Could you check a few things on this model? Use its own coordinates, in mm. A direction names the side the tool comes from. Give positions to 0.01 mm unless a question says otherwise; leave off trailing zeros. Write each loop counter-clockwise with the first axis right and the second up, starting at its lowest first coordinate (ties: lowest second). Pieces come first, ordered by that corner, then holes. Notation, with made-up numbers: (4, 37.25) -> (28, 37.25) arc R23 ccw to (28, 67.25) -> close; hole circle Ø7 at (23.25, 13.25). An arc over 180 degrees is marked (long way). Write item = value, one per line. Start each with the question number.
```python
from build123d import *

# Parameters (mm, degrees)
SKETCH1_W                                           = 97
SKETCH1_H                                           = 32.5
BOSS_EXTRUDE1_DEPTH                                 = 6
SKETCH5_R                                           = 20
BOSS_EXTRUDE5_DEPTH                                 = 20
CBORE_FOR_M5_HEX_SOCKET_HEAD_CAP_SCREW1_D           = 5.5
CBORE_FOR_M5_HEX_SOCKET_HEAD_CAP_SCREW1_CBORE_D     = 10
CBORE_FOR_M5_HEX_SOCKET_HEAD_CAP_SCREW1_CBORE_DEPTH = 5.9
SKETCH16_R                                          = 2.5
BOSS_EXTRUDE6_DEPTH                                 = 5
BOSS_EXTRUDE7_START                                 = -27.5
SKETCH16_2_R                                        = 2.5
BOSS_EXTRUDE7_DEPTH                                 = 5
SKETCH17_R                                          = 5
CUT_EXTRUDE3_DEPTH                                  = 3
SKETCH18_R                                          = 5
SKETCH18_R_2                                        = 2.75
BOSS_EXTRUDE8_DEPTH                                 = 2.9
CUT_EXTRUDE4_DEPTH                                  = 20


with BuildPart() as part:
    # Sketch1 → Boss-Extrude1 (new body)
    with BuildSketch(Plane(origin=(0, 0, 0), x_dir=(1, 0, 0), z_dir=(0, 1, 0))):
        with Locations((48.5, 16.25)):
            Rectangle(SKETCH1_W, SKETCH1_H)
    extrude(amount=BOSS_EXTRUDE1_DEPTH)

    # Sketch5 → Boss-Extrude5 (add)
    with BuildSketch(Plane(origin=(0, 6, 0), x_dir=(1, 0, 0), z_dir=(0, 1, 0))):
        with Locations(Location((48.5, 16.25, 0), (0, 0, 54.340912304))):
            Circle(SKETCH5_R)
    extrude(amount=BOSS_EXTRUDE5_DEPTH)

    # CBORE for M5 Hex Socket Head Cap Screw1 (through all)
    with Locations(Plane.XZ):
        with Locations((37.363068196, -5.113068196), (59.636931804, -5.113068196), (59.636931804, -27.386931804), (37.363068196, -27.386931804)):
            CounterBoreHole(CBORE_FOR_M5_HEX_SOCKET_HEAD_CAP_SCREW1_D / 2, CBORE_FOR_M5_HEX_SOCKET_HEAD_CAP_SCREW1_CBORE_D / 2, CBORE_FOR_M5_HEX_SOCKET_HEAD_CAP_SCREW1_CBORE_DEPTH)

    # Sketch16 → Boss-Extrude6 (add)
    # profile 1 of 2: a face of its own
    with BuildSketch(Plane.XY):
        with BuildLine():
            Line((87, 6), (77, 6))
            Line((77, 6), (77, 13))
            ThreePointArc((77, 13), (77.585786438, 14.414213562), (79, 15))
            Line((79, 15), (85, 15))
            ThreePointArc((85, 15), (86.414213562, 14.414213562), (87, 13))
            Line((87, 13), (87, 6))
        make_face()
        with Locations(Location((82, 11.5, 0), (0, 0, 180))):
            Circle(SKETCH16_R, mode=Mode.SUBTRACT)
    # profile 2 of 2: a face of its own
    with BuildSketch(Plane.XY):
        with BuildLine():
            Line((10, 6), (10, 13))
            ThreePointArc((10, 13), (10.585786438, 14.414213562), (12, 15))
            Line((12, 15), (18, 15))
            ThreePointArc((18, 15), (19.414213562, 14.414213562), (20, 13))
            Line((20, 13), (20, 6))
            Line((20, 6), (10, 6))
        make_face()
        with Locations((15, 11.5)):
            Circle(SKETCH16_R, mode=Mode.SUBTRACT)
    extrude(amount=-BOSS_EXTRUDE6_DEPTH)

    # Sketch16<2> → Boss-Extrude7 (add)
    # profile 1 of 2: a face of its own
    with BuildSketch(Plane.XY.offset(BOSS_EXTRUDE7_START)):
        with BuildLine():
            Line((87, 6), (77, 6))
            Line((77, 6), (77, 13))
            ThreePointArc((77, 13), (77.585786438, 14.414213562), (79, 15))
            Line((79, 15), (85, 15))
            ThreePointArc((85, 15), (86.414213562, 14.414213562), (87, 13))
            Line((87, 13), (87, 6))
        make_face()
        with Locations(Location((82, 11.5, 0), (0, 0, 180))):
            Circle(SKETCH16_2_R, mode=Mode.SUBTRACT)
    # profile 2 of 2: a face of its own
    with BuildSketch(Plane.XY.offset(BOSS_EXTRUDE7_START)):
        with BuildLine():
            Line((10, 6), (10, 13))
            ThreePointArc((10, 13), (10.585786438, 14.414213562), (12, 15))
            Line((12, 15), (18, 15))
            ThreePointArc((18, 15), (19.414213562, 14.414213562), (20, 13))
            Line((20, 13), (20, 6))
            Line((20, 6), (10, 6))
        make_face()
        with Locations((15, 11.5)):
            Circle(SKETCH16_2_R, mode=Mode.SUBTRACT)
    extrude(amount=-BOSS_EXTRUDE7_DEPTH)

    # Sketch17 → Cut-Extrude3 (cut)
    # profile 1 of 8: a face of its own
    with BuildSketch(Plane.XZ):
        with BuildLine():
            ThreePointArc((42.863068196, -27.386931804), (37.363068196, -21.886931804), (31.863068196, -27.386931804))
            Line((31.863068196, -27.386931804), (31.863068196, -32.5))
            Line((31.863068196, -32.5), (42.863068196, -32.5))
            Line((42.863068196, -32.5), (42.863068196, -27.386931804))
        make_face()
        with Locations(Location((37.363068196, -27.386931804, 0), (0, 0, 270))):
            Circle(SKETCH17_R, mode=Mode.SUBTRACT)
    # profile 2 of 8: a face of its own
    with BuildSketch(Plane.XZ):
        with BuildLine():
            Line((54.136931804, -27.386931804), (54.136931804, -32.5))
            Line((54.136931804, -32.5), (65.136931804, -32.5))
            Line((65.136931804, -32.5), (65.136931804, -27.386931804))
            ThreePointArc((65.136931804, -27.386931804), (59.636931804, -21.886931804), (54.136931804, -27.386931804))
        make_face()
        with Locations(Location((59.636931804, -27.386931804, 0), (0, 0, 270))):
            Circle(SKETCH17_R, mode=Mode.SUBTRACT)
    # profile 3 of 8: a face of its own
    with BuildSketch(Plane.XZ):
        with BuildLine():
            Line((54.136931804, 0), (54.136931804, -5.113068196))
            ThreePointArc((54.136931804, -5.113068196), (59.636931804, -10.613068196), (65.136931804, -5.113068196))
            Line((65.136931804, -5.113068196), (65.136931804, 0))
            Line((65.136931804, 0), (54.136931804, 0))
        make_face()
        with Locations(Location((59.636931804, -5.113068196, 0), (0, 0, 270))):
            Circle(SKETCH17_R, mode=Mode.SUBTRACT)
    # profile 4 of 8: a face of its own
    with BuildSketch(Plane.XZ):
        with BuildLine():
            Line((42.863068196, -5.113068196), (42.863068196, 0))
            Line((42.863068196, 0), (31.863068196, 0))
            Line((31.863068196, 0), (31.863068196, -5.113068196))
            ThreePointArc((31.863068196, -5.113068196), (37.363068196, -10.613068196), (42.863068196, -5.113068196))
        make_face()
        with Locations(Location((37.363068196, -5.113068196, 0), (0, 0, 270))):
            Circle(SKETCH17_R, mode=Mode.SUBTRACT)
    # profile 5 of 8: a face of its own
    with BuildSketch(Plane.XZ):
        with Locations(Location((37.363068196, -27.386931804, 0), (0, 0, 270))):
            Circle(SKETCH17_R)
    # profile 6 of 8: a face of its own
    with BuildSketch(Plane.XZ):
        with Locations(Location((59.636931804, -27.386931804, 0), (0, 0, 270))):
            Circle(SKETCH17_R)
    # profile 7 of 8: a face of its own
    with BuildSketch(Plane.XZ):
        with Locations(Location((59.636931804, -5.113068196, 0), (0, 0, 270))):
            Circle(SKETCH17_R)
    # profile 8 of 8: a face of its own
    with BuildSketch(Plane.XZ):
        with Locations(Location((37.363068196, -5.113068196, 0), (0, 0, 270))):
            Circle(SKETCH17_R)
    extrude(amount=-CUT_EXTRUDE3_DEPTH, mode=Mode.SUBTRACT)

    # Sketch18 → Boss-Extrude8 (add)
    # profile 1 of 4: a face of its own
    with BuildSketch(Plane.XZ.offset(-5.9)):
        with Locations((37.363068196, -27.386931804)):
            Circle(SKETCH18_R)
        with Locations(Location((37.363068196, -27.386931804, 0), (0, 0, 270))):
            Circle(SKETCH18_R_2, mode=Mode.SUBTRACT)
    # profile 2 of 4: a face of its own
    with BuildSketch(Plane.XZ.offset(-5.9)):
        with Locations((37.363068196, -5.113068196)):
            Circle(SKETCH18_R)
        with Locations(Location((37.363068196, -5.113068196, 0), (0, 0, 270))):
            Circle(SKETCH18_R_2, mode=Mode.SUBTRACT)
    # profile 3 of 4: a face of its own
    with BuildSketch(Plane.XZ.offset(-5.9)):
        with Locations((59.636931804, -5.113068196)):
            Circle(SKETCH18_R)
        with Locations(Location((59.636931804, -5.113068196, 0), (0, 0, 270))):
            Circle(SKETCH18_R_2, mode=Mode.SUBTRACT)
    # profile 4 of 4: a face of its own
    with BuildSketch(Plane.XZ.offset(-5.9)):
        with Locations((59.636931804, -27.386931804)):
            Circle(SKETCH18_R)
        with Locations(Location((59.636931804, -27.386931804, 0), (0, 0, 270))):
            Circle(SKETCH18_R_2, mode=Mode.SUBTRACT)
    extrude(amount=BOSS_EXTRUDE8_DEPTH)

    # Sketch19 → Cut-Extrude4 (cut)
    with BuildSketch(Plane.XZ.offset(-6)):
        with BuildLine():
            Line((36.840776184, 0), (60.159223816, 0))
            ThreePointArc((60.159223816, 0), (48.5, 3.75), (36.840776184, 0))
        make_face()
        with BuildLine():
            Line((60.159223816, -32.5), (36.840776184, -32.5))
            ThreePointArc((36.840776184, -32.5), (48.5, -36.25), (60.159223816, -32.5))
        make_face()
    extrude(amount=-CUT_EXTRUDE4_DEPTH, mode=Mode.SUBTRACT)


solid = part.part
```
(1) On a 3-axis mill with a long thin cutter (end or side, diameter ignored), from which of +Z, -Z, +X, -X, +Y, -Y can I reach the whole of each face in a straight line? I mean faces 1 (the flat face through (42.863, 1, -30)), 2 (the flat face through (15.1, 8.6, -27.5)), 3 (the flat face through (82, 15, -2)), 4 (the cylindrical face through (68.5, 15.9, -16)). Say none if no direction works.
(2) If I drill on line 1 along Z through (x, y) = (17.5, 11); line 2 along X through (y, z) = (17.25, -4); line 3 along X through (y, z) = (21.5, -3), over which ranges is the centre line in solid material (lowest first)? Write a range as from..to.
(3) Imagine slicing it at B-B (y = 11.5). State how many separate pieces and enclosed holes the cut face has, then the cut area to 3 significant figures.
(4) Imagine slicing it at A-A (x = 82). Please give me the cut outline in (y, z), then the cut area to 3 significant figures.
(5) I'm going to push flat-ended pins straight in: pin 1 (4 mm diameter, centred on y = 11, z = -29.5, fed in from -X); pin 2 (3 mm diameter, centred on x = 82, y = 11.5, fed in from +Z); pin 3 (3 mm diameter, centred on x = 73.5, z = -8.5, fed in from -Y); pin 4 (3 mm diameter, centred on x = 57.5, z = -27, fed in from -Y). Where does each tip first touch, or does it pass through?
(6) We'd pull the mould along Y, two halves only. Please class faces 5 (the flat face through (54.137, 1, -30)), 6 (the cylindrical face through (13, 10, -2)), 7 (the cylindrical face through (77.57, 14.4, -2.46)): released by +Y, released by -Y, zero draft, split by the parting line, or undercut.
(7) Imagine slicing it at D-D (z = -19.5). Please give me the cut outline in (x, y).
Answers below:
q1.face_1 = -Z, -Y
q1.face_2 = -X, +Y
q1.face_3 = +Z, -Z, +X, +Y
q1.face_4 = +Y
q2.line_1 = -32.5..-27.5, -5..0
q2.line_2 = 32.69..34.85, 39.88..57.12, 62.15..64.31
q2.line_3 = 33.52..35.6, 39.12..57.88, 61.4..63.48
q3.separate_pieces = 9
q3.enclosed_holes = 4
q3.area = 1,140 mm^2
q4.outline = (0, -32.5) -> (9, -32.5) -> (9, -27.5) -> (6, -27.5) -> (6, -5) -> (9, -5) -> (9, 0) -> (0, 0) -> close; (14, -32.5) -> (15, -32.5) -> (15, -27.5) -> (14, -27.5) -> close; (14, -5) -> (15, -5) -> (15, 0) -> (14, 0) -> close
q4.area = 235 mm^2
q5.pin_1 = 10
q5.pin_2 = through
q5.pin_3 = 0
q5.pin_4 = 3
q6.face_5 = zero draft
q6.face_6 = undercut
q6.face_7 = released by +Y
q7.outline = (0, 0) -> (97, 0) -> (97, 6) -> (68.23, 6) -> (68.23, 26) -> (28.77, 26) -> (28.77, 6) -> (0, 6) -> close
